Autodesk Inventor part; units mm, degrees
ref_plane "YZ Plane" through (0, 0, 0) normal (1, 0, 0) x (0, 1, 0)
ref_plane "XZ Plane" through (0, 0, 0) normal (0, 1, 0) x (-1, 0, 0)
ref_plane "XY Plane" through (0, 0, 0) normal (0, 0, 1) x (1, 0, 0)
sketch "Sketch1" plane through (0, 0, 0) normal (0, 0, 1) x (1, 0, 0)
  line L0 (0, 0) -> (200, 0)
  line L1 (200, 0) -> (200, 260)
  line L2 (200, 260) -> (0, 260)
  line L3 (0, 260) -> (0, 0)
  dimension "d0" = 200
  dimension "d1" = 260
extrude "Extrusion1" add sketch "Sketch1" along normal blind 20
sketch "Sketch2" plane through (0, 0, 20) normal (0, 0, 1) x (1, 0, 0)
  circle A0 centre (100, 160) radius 42.5
  line L0 (200, 260) -> (0, 260)
  line L1 (0, 260) -> (0, 0)
  dimension "d4" = 85
  dimension "d5" = 100
  dimension "d6" = 100
extrude "Extrusion2" cut sketch "Sketch2" against normal blind 20
sketch "Sketch3" plane through (0, 0, 0) normal (0, 0, -1) x (-1, 0, 0)
  circle A0 centre (-150, 12.5) radius 6.35
  circle A1 centre (-50, 12.5) radius 6.35
  line L0 (0, 0) -> (-200, 0)
  line L1 (-200, 0) -> (-200, 260)
  line L2 (0, 260) -> (0, 0)
  dimension "d9" = 12.7
  dimension "d10" = 12.7
  dimension "d11" = 12.5
  dimension "d12" = 12.5
  dimension "d13" = 50
  dimension "d14" = 50
extrude "Extrusion3" cut sketch "Sketch3" against normal blind 20
equation "\"d12\" = d11"
equation "\"d14\" = d13"
properties part number "FloorMountFacePlate"
CAD build for the part. Positions are in the model's coordinates, mm. Coordinates: 2 decimals unless noted, no trailing zeros. Write each loop counter-clockwise with the first axis right and the second up, starting at its lowest first coordinate (ties: lowest second). Pieces come first, ordered by that corner, then holes. Notation, with made-up numbers: (-30, 8) -> (-24, 8) arc R25 cw to (-24, 46) -> close; hole circle Ø2 at (-7.5, -27). An arc over 180 degrees is marked (long way). Use CSV: the item, a comma, the result in double quotes. Start each with the question number.
Item 1: Wall check: probe 1 along Y at (x, z) = (150, 10.5); probe 2 along Y at (x, z) = (100, 9.5); probe 3 along X at (y, z) = (176.5, 14.25). Give the ranges that are in metal, low to high.
Item 2: Band-saw the part on B-B, the plane y = 160. Write the cut outline in (x, z).
Item 3: Band-saw the part on A-A, the plane x = 100. Write the cut outline in (y, z), plus the area to 3 significant figures.
Item 4: Band-saw the part on D-D, the plane y = 12.5. Write the cut outline in (x, z).
Item 5: Drop flat-ended pins along their axis: P1, Ø1, axis at x = 158, z = 14, coming from the -Y side; P2, Ø7.5, axis at x = 150, y = 12.5, coming from the -Z side. Give the stop position or say it passes through.
Item 6: Band-saw the part on C-C, the plane z = 5. Write the cut outline in (x, y), plus the area to 3 significant figures.
Item 7: Two-plate mould, pull along Y, no slides. Class faces 1 (the cylindrical face through (56.344, 12.779, 9.86)), 2 (the flat face through (0, 132, 10)), 3 (the flat face through (101, 260, 10)), 4 (the flat face through (99, 0, 10)): +Y half, -Y half, draft (parallel to the pull), parting line (faces both ways), or undercut.
Response values:
1,probe 1,"y = 0 to 6.15, 18.85 to 260"
1,probe 2,"y = 0 to 117.5, 202.5 to 260"
1,probe 3,"x = 0 to 60.83, 139.17 to 200"
2,outline,"(0, 0) -> (57.5, 0) -> (57.5, 20) -> (0, 20) -> close; (142.5, 0) -> (200, 0) -> (200, 20) -> (142.5, 20) -> close"
3,outline,"(0, 0) -> (117.5, 0) -> (117.5, 20) -> (0, 20) -> close; (202.5, 0) -> (260, 0) -> (260, 20) -> (202.5, 20) -> close"
3,area,"3,500 mm2"
4,outline,"(0, 0) -> (43.65, 0) -> (43.65, 20) -> (0, 20) -> close; (56.35, 0) -> (143.65, 0) -> (143.65, 20) -> (56.35, 20) -> close; (156.35, 0) -> (200, 0) -> (200, 20) -> (156.35, 20) -> close"
5,P1,"stops at y = 0"
5,P2,"passes through"
6,outline,"(0, 0) -> (200, 0) -> (200, 260) -> (0, 260) -> close; hole circle Ø12.7 at (50, 12.5); hole circle Ø85 at (100, 160); hole circle Ø12.7 at (150, 12.5)"
6,area,"46,100 mm2"
7,face 1,"undercut"
7,face 2,"draft"
7,face 3,"+Y half"
7,face 4,"-Y half"
